```python
from build123d import *

# Parameters (mm, degrees)
SKETCH_1_R          = 6
EXTRUDE_1_DEPTH     = 35
EXTRUDE_2_DEPTH     = 7.5
SKETCH_3_R          = 3.75
EXTRUDE_3_DEPTH     = 10
CHAMFER_1_SIZE      = 0.5
CHAMFER_2_SIZE      = 0.5
SKETCH_5_W          = 3
SKETCH_5_H          = 3
CUT_EXTRUDE_1_DEPTH = 10
FILLET_1_R          = 1.5
FILLET_2_R          = 0.5


with BuildPart() as part:
    # 草图1 → 凸台-拉伸1 (new body)
    with BuildSketch(Plane.XY):
        Circle(SKETCH_1_R)
    extrude(amount=-EXTRUDE_1_DEPTH)

    # 草图2 → 凸台-拉伸2 (add)
    with BuildSketch(Plane.XY):
        with BuildLine():
            Line((9.637888197, -2.666666667), (5.782732918, -16.6))
            ThreePointArc((5.782732918, -16.6), (0, -21), (-5.782732918, -16.6))
            Line((-5.782732918, -16.6), (-9.637888197, -2.666666667))
            ThreePointArc((-9.637888197, -2.666666667), (0, 10), (9.637888197, -2.666666667))
        make_face()
    extrude(amount=EXTRUDE_2_DEPTH)

    # 草图3 → 凸台-拉伸3 (add)
    with BuildSketch(Plane.XY.offset(7.5)):
        with Locations((0, -15)):
            Circle(SKETCH_3_R)
    extrude(amount=EXTRUDE_3_DEPTH)

    # 倒角1
    chamfer_1_edges = [part.edges().sort_by_distance(p)[0] for p in [
        (-3.75, -15, 17.5),
    ]]
    chamfer(chamfer_1_edges, length=CHAMFER_1_SIZE)

    # 倒角2
    chamfer_2_edges = [part.edges().sort_by_distance(p)[0] for p in [
        (-6, 0, -35),
    ]]
    chamfer(chamfer_2_edges, length=CHAMFER_2_SIZE)

    # 草图5 → 切除-拉伸1 (cut)
    with BuildSketch(Plane(origin=(0, 0, -35), x_dir=(-1, 0, 0), z_dir=(0, 0, -1))):
        with Locations((0, 6)):
            Rectangle(SKETCH_5_W, SKETCH_5_H)
    extrude(amount=-CUT_EXTRUDE_1_DEPTH, mode=Mode.SUBTRACT)

    # 圆角1
    fillet_1_edges = [part.edges().sort_by_distance(p)[0] for p in [
        (-1.5, 5.15473751, -25),
        (1.5, 5.15473751, -25),
    ]]
    fillet(fillet_1_edges, radius=FILLET_1_R - 0.0001)  # a hair under: the kernel refuses the full size

    # 圆角2
    fillet_2_edges = [part.edges().sort_by_distance(p)[0] for p in [
        (0, -21, 0),
        (7.710310557, -9.633333333, 0),
        (0, 10, 0),
        (-7.710310557, -9.633333333, 0),
        (0, -21, 7.5),
        (7.710310557, -9.633333333, 7.5),
        (0, 10, 7.5),
        (-7.710310557, -9.633333333, 7.5),
    ]]
    fillet(fillet_2_edges, radius=FILLET_2_R)


solid = part.part
```
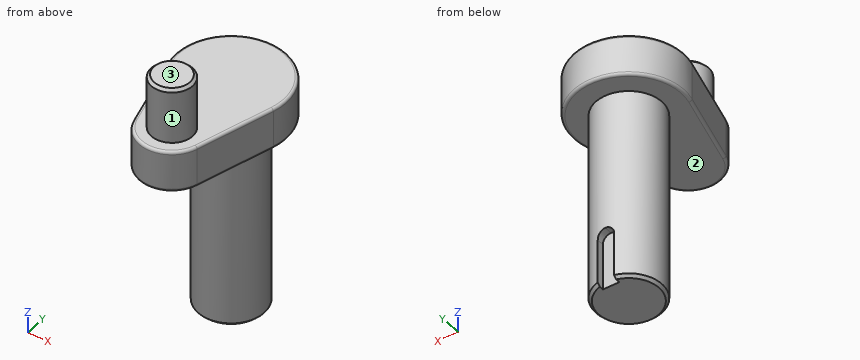
Model file for the job. Use its own axes, mm. Face numbers are marked on the shaded views. A direction names the side the tool comes from. Coordinates: 2 decimals unless noted, no trailing zeros. Order: outer loops, then holes, each group sorted by start corner. A loop starts at its lowest first (then second) coordinate and runs counter-clockwise, first axis right, second up. Notation, with made-up numbers: (38.25, 15.5) - (75.25, 15.5) arc R33 cw to (75.25, 43.5) - close; hole circle Ø1 at (25, 46). An arc over 180 degrees is marked (long way). Return JSON: item names as keys, results as strings. Group by question number.
1) Flat gauge pins, fed straight in: P1, Ø0.7, axis at y = 5.5, z = -31, coming from the -X side; P2, Ø3.5, axis at x = 0.5, z = -30, coming from the +Y side; P3, Ø1.4, axis at y = 5, z = -30, coming from the +X side. Where does each tip first touch, or does it go through?
2) Tool access for the marked faces 1, 2 and 3: list every direction of +Z, -Z, +X, -X, +Y, -Y with a clear straight run to the whole face (end or side of a thin tool).
3) Saw through at B-B, the plane z = -20.5. Write the cut outline in (x, y), plus the area to 3 significant figures.
4) Probe line 1 (Z direction, x = 5, y = 7); line 2 (Z direction, x = 5, y = 2); line 3 (Y direction, x = -3.25, z = 11.5). List the from-to ranges inside material, lowest first. Write a range as from..to.
5) Saw through at A-A, the plane z = -30. Write the cut outline in (x, y), plus the area to 3 significant figures.
Values found:
{
 "1": {"P1": "stops at x = -3.08", "P2": "stops at y = 5.81", "P3": "stops at x = 4.18"},
 "2": {"face 1": "+Z", "face 2": "-Z", "face 3": "+Z, +X, -X, +Y, -Y"},
 "3": {"outline": "circle Ø12 at (0, 0)", "area": "113 mm²"},
 "4": {"line 1": "z = 0..7.5", "line 2": "z = -35..7.5", "line 3": "y = -16.87..-13.13"},
 "5": {"outline": "(-1.5, 4.5) - (-1.5, 5.81) arc R6 ccw (long way) to (1.5, 5.81) - (1.5, 4.5) - close", "area": "109 mm²"}
}
